from build123d import *

# Parameters (mm, degrees)
EXTRUDE_1_DEPTH              = 2.9
SKETCH_2_R                   = 3.5
EXTRUDE_2_DEPTH              = 5
FILLET_1_R                   = 1
FILLET_2_R                   = 0.2
HOLE_WIZARD_M4_1_D           = 3.3
HOLE_WIZARD_M4_1_DEPTH       = 10.1
HOLE_WIZARD_M4_1_CSINK_D     = 4.05
HOLE_WIZARD_M4_1_CSINK_ANGLE = 90
HOLE_WIZARD_M4_1_TIP         = 0.991420021


with BuildPart() as part:
    # 草图1 → 凸台-拉伸1 (new body)
    with BuildSketch(Plane(origin=(0, 0, 0), x_dir=(1, 0, 0), z_dir=(0, 1, 0))):
        Polygon((3.5, -2.020725942), (3.5, 2.020725942), (0, 4.041451884), (-3.5, 2.020725942), (-3.5, -2.020725942), (0, -4.041451884), align=None)
    extrude(amount=EXTRUDE_1_DEPTH)

    # 草图2 → 凸台-拉伸2 (add)
    with BuildSketch(Plane.XZ):
        Circle(SKETCH_2_R)
    extrude(amount=-EXTRUDE_2_DEPTH)

    # 圆角1
    fillet_1_edges = [part.edges().sort_by_distance(p)[0] for p in [
        (-3.5, 5, 0),
    ]]
    fillet(fillet_1_edges, radius=FILLET_1_R)

    # 圆角2
    fillet_2_edges = [part.edges().sort_by_distance(p)[0] for p in [
        (0, 1.45, 4.041451884),
        (-3.5, 1.45, 2.020725942),
        (-3.5, 1.45, -2.020725942),
        (0, 1.45, -4.041451884),
        (3.5, 1.45, -2.020725942),
        (3.5, 1.45, 2.020725942),
    ]]
    fillet(fillet_2_edges, radius=FILLET_2_R)

    # M4 螺纹孔1
    with Locations(Plane(origin=(0, 0, 0), x_dir=(-1, 0, 0), z_dir=(0, -1, 0))):
        with Locations((0, 0)):
            CounterSinkHole(HOLE_WIZARD_M4_1_D / 2, HOLE_WIZARD_M4_1_CSINK_D / 2, depth=HOLE_WIZARD_M4_1_DEPTH, counter_sink_angle=HOLE_WIZARD_M4_1_CSINK_ANGLE)
            with Locations((0, 0, -(HOLE_WIZARD_M4_1_DEPTH + HOLE_WIZARD_M4_1_TIP / 2))):  # 118° drill point
                Cone(0, HOLE_WIZARD_M4_1_D / 2, HOLE_WIZARD_M4_1_TIP, mode=Mode.SUBTRACT)


solid = part.part
Read the model definition and answer for the solid it produces. Units are mm, in the model's axes. A direction names the side the tool comes from. Round coordinates to 2 decimals unless told otherwise and drop trailing zeros. Loops run counter-clockwise (first coordinate to the right, second up) from the corner with the lowest first, then second, coordinate; pieces in that order, holes last.
Q1. Section C-C on y = 3.9 is taken. Write down the section's boundary in (x, z), and give its area (3 significant figures).
Q2. Section A-A on x = 0 is taken. Write down the section's boundary in (y, z) (3 decimals), and give its area (3 significant figures).
Q3. Each of these flat-tipped pins is pushed along its axis until it touches: pin 1 (2 mm diameter, centred on y = 3.5, z = -1.5, fed in from -X); pin 2 (0.9 mm diameter, centred on x = 3, z = 2, fed in from +Y); pin 3 (2 mm diameter, centred on x = 0, z = 0, fed in from -Y); pin 4 (1.5 mm diameter, centred on x = -2, y = 1.5, fed in from +Z). Where does it stop, or does it pass through?
Q4. Determine the mould class of faces 1 (the face through (-1.216, 2.72, -1.115)), 2 (the face through (-3.15, 2.9, 1.85)), 3 (the face through (1.727, 1.43, 3.044)) for opening direction Z: released by +Z, released by -Z, zero draft, split by the parting line, or undercut.
Q5. Section D-D on y = 4.65 is taken. Write down the section's boundary in (x, z), and give its area (3 significant figures).
Q6. Consider probe 1 along Z at (x, y) = (0, 1.5); probe 2 along Z at (x, y) = (0, 3.5); probe 3 along Z at (x, y) = (1.75, 2.95). Determine where each line is inside the solid, lowest interval first.
Q7. Section B-B on y = 0.75 is taken. Write down the section's boundary in (x, z), and give its area (3 significant figures).
Q8. Which of the six approach directions +Z, -Z, +X, -X, +Y, -Y give full straight-line access (tool end or side, diameter ignored) to faces 4 (the face through (3.233, 3.442, -1.341)), 5 (the face through (3.2, 2.9, 1.8)), 6 (the face through (-3.15, 2.9, -1.86))?
Output:
1. outline: circle Ø7 at (0, 0); hole circle Ø3.3 at (0, 0)
1. area: 29.9 mm2
2. outline: (0, -4.011) - (2.9, -4.011) - (2.9, -3.5) - (4, -3.5) arc R1 ccw to (5, -2.5) - (5, -1.65) - (0.375, -1.65) - (0, -2.025) - close; (0, 2.025) - (0.375, 1.65) - (5, 1.65) - (5, 2.5) arc R1 ccw to (4, 3.5) - (2.9, 3.5) - (2.9, 4.011) - (0, 4.011) - close
2. area: 20.9 mm2
3. pin 1: stops at x = -3.5
3. pin 2: stops at y = 4.76
3. pin 3: passes through
3. pin 4: stops at z = 3.32
4. face 1: undercut
4. face 2: zero draft
4. face 3: released by +Z
5. outline: circle Ø6.52 at (0, 0); hole circle Ø3.3 at (0, 0)
5. area: 24.8 mm2
6. probe 1: z = -4.01 to -1.65, 1.65 to 4.01
6. probe 2: z = -3.5 to -1.65, 1.65 to 3.5
6. probe 3: z = -3.03 to 3.03
7. outline: (-3.5, -1.91) arc R0.2 ccw to (-3.4, -2.08) - (-0.1, -3.98) arc R0.2 ccw to (0.1, -3.98) - (3.4, -2.08) arc R0.2 ccw to (3.5, -1.91) - (3.5, 1.91) arc R0.2 ccw to (3.4, 2.08) - (0.1, 3.98) arc R0.2 ccw to (-0.1, 3.98) - (-3.4, 2.08) arc R0.2 ccw to (-3.5, 1.91) - close; hole circle Ø3.3 at (0, 0)
7. area: 33.9 mm2
8. face 4: +Y
8. face 5: +Z, +X, +Y
8. face 6: -Z, -X, +Y
